Geometry check sheet. Reference: the model listing, model coordinates, mm. Round coordinates to 2 decimals unless told otherwise and drop trailing zeros. Order: outer loops, then holes, each group sorted by start corner. A loop starts at its lowest first (then second) coordinate and runs counter-clockwise, first axis right, second up.
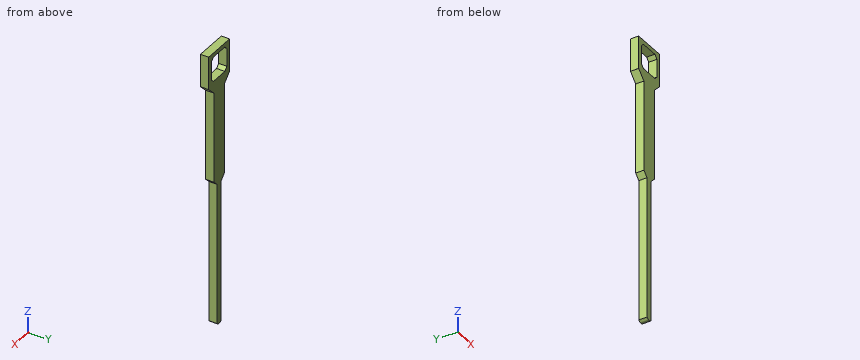
```python
from build123d import *

# Parameters (mm, degrees)
F0_W        = 5.08
F0_H        = 114.3
F1_DEPTH    = 6.35
F2_SIZE     = 1.27
F3_R        = 2.54
F4_T1_DEPTH = 6.35
F4_T6_DEPTH = 6.35
F5_SIZE     = 2.54
F6_T1_DEPTH = 6.35
F6_T6_DEPTH = 6.35


# Not quite as in the source:
# - a fillet or chamfer that OpenCascade refuses, or shapes differently, is made with other operations: its cross-section is extruded or revolved along the edge and cut away or added


with BuildPart() as f1:
    # F0 (on Front) → F1 (new body)
    with BuildSketch(Plane.XZ):
        Polygon((12.7, 38.1), (12.7, 63.5), (-12.7, 63.5), (-12.7, 38.1), (-6.3373190351, 38.1), (-6.3373190351, -38.1), (-2.54, -38.1), (2.54, -38.1), (6.3626809649, -38.1), (6.3626809649, 38.1), align=None)
        Polygon((-9.5123190351, 60.325), (9.5376809649, 60.325), (9.5376809649, 41.275), (6.3626809649, 41.275), (-6.3373190351, 41.275), (-9.5123190351, 41.275), align=None, mode=Mode.SUBTRACT)
        with Locations((0, -95.25)):
            Rectangle(F0_W, F0_H)
    extrude(amount=F1_DEPTH)

    # F2
    f2_edges = [f1.edges().sort_by_distance(p)[0] for p in [
        (-2.54, -3.175, -152.4),
        (2.54, -3.175, -152.4),
    ]]
    chamfer(f2_edges, length=F2_SIZE)

    # F3
    f3_edges = [f1.edges().sort_by_distance(p)[0] for p in [
        (-1.27, -3.175, -152.4),
        (1.27, -3.175, -152.4),
    ]]
    fillet(f3_edges, radius=F3_R)

    # F4: chamfer of 3.81 on 2 edges, made by hand

    # F4_s2 → F4_t1 (join)
    with BuildSketch(Plane.XZ):
        Polygon((2.54, -41.91), (6.35, -38.1), (2.54, -38.1), align=None)
    extrude(amount=F4_T1_DEPTH)


with BuildPart() as f4_tool4:
    # F4_s5 → F4_t6 (new body)
    with BuildSketch(Plane.XZ):
        Polygon((-2.54, -41.91), (-6.35, -38.1), (-2.54, -38.1), align=None)
    extrude(amount=F4_T6_DEPTH)

    split(bisect_by=Plane.YZ.offset(-6.3373190351), keep=Keep.TOP)


with BuildPart() as f1_1:
    add(f1.part)

    # F4_t3: union F4_tool4
    add(f4_tool4.part)

    # F5
    f5_edges = [f1_1.edges().sort_by_distance(p)[0] for p in [
        (-9.512319, -3.175, 60.325),
        (9.537681, -3.175, 60.325),
        (-9.512319, -3.175, 41.275),
        (9.537681, -3.175, 41.275),
    ]]
    chamfer(f5_edges, length=F5_SIZE)

    # F6: chamfer of 6.35 on 2 edges, made by hand

    # F6_s2 → F6_t1 (join)
    with BuildSketch(Plane.XZ):
        Polygon((-12.6873190351, 38.1), (-6.3373190351, 31.75), (-6.3373190351, 38.1), align=None)
    extrude(amount=F6_T1_DEPTH)


with BuildPart() as f6_tool4:
    # F6_s5 → F6_t6 (new body)
    with BuildSketch(Plane.XZ):
        Polygon((6.3626809649, 31.75), (12.7126809649, 38.1), (6.3626809649, 38.1), align=None)
    extrude(amount=F6_T6_DEPTH)

    split(bisect_by=Plane.YZ.offset(12.7), keep=Keep.BOTTOM)


with BuildPart() as f1_2:
    add(f1_1.part)

    # F6_t3: union F6_tool4
    add(f6_tool4.part)


solid = f1_2.part
```
(1) Material ranges on line 1 (X direction, y = -5.25, z = 54.5); line 2 (Z direction, x = 2.5, y = -5) (3 decimals); line 3 (X direction, y = -5.25, z = -2), recorded low to high.
Returned:
line 1: x = -12.7 to -9.51, 9.54 to 12.7
line 2: z = -151.17 to 41.275, 60.325 to 63.5
line 3: x = -6.34 to 6.36
(2) Sectioned sample at C-C, the plane z = 26.5. Record the cut outline in (x, y).
Returned:
outline: (-6.34, -6.35) - (6.36, -6.35) - (6.36, 0) - (-6.34, 0) - close
(3) Depth check by flat-ended pin: P1, Ø3, axis at y = -1.5, z = -109.5, coming from the -X side; P2, Ø1, axis at y = -1, z = -53, coming from the +X side; P3, Ø1, axis at y = -1.5, z = 20, coming from the +X side. Enter the tip coordinate at first touch or a pass-through.
Returned:
P1: stops at x = -2.54
P2: stops at x = 2.54
P3: stops at x = 6.36
(4) Sectioned sample at A-A, the plane y = -2.5. Record the cut outline in (x, z) (3 decimals).
Returned:
outline: (-12.7, 38.1) - (-12.687, 38.1) - (-6.337, 31.75) - (-6.337, -38.113) - (-2.54, -41.91) - (-2.54, -151.13) - (-2.014, -151.656) arc R2.54 ccw to (-0.218, -152.4) - (0.218, -152.4) arc R2.54 ccw to (2.014, -151.656) - (2.54, -151.13) - (2.54, -41.91) - (6.35, -38.1) - (6.363, -38.1) - (6.363, 31.75) - (12.7, 38.087) - (12.7, 63.5) - (-12.7, 63.5) - close; hole (-9.512, 43.815) - (-6.972, 41.275) - (6.998, 41.275) - (9.538, 43.815) - (9.538, 57.785) - (6.998, 60.325) - (-6.972, 60.325) - (-9.512, 57.785) - close
(5) Sectioned sample at B-B, the plane z = -49.5. Record the cut outline in (x, y), and give its area (3 significant figures).
Returned:
outline: (-2.54, -6.35) - (2.54, -6.35) - (2.54, 0) - (-2.54, 0) - close
area: 32.3 mm2
